Check sheet for the modelled part. Datum: model origin and axes. Units: mm. A direction names the side the tool comes from. Coordinates: 2 decimals unless noted, no trailing zeros. Order: outer loops, then holes, each group sorted by start corner. A loop starts at its lowest first (then second) coordinate and runs counter-clockwise, first axis right, second up.
from build123d import *

# Parameters (mm, degrees)
PAD_DEPTH        = 55.5
HOLE_D           = 4
HOLE_DEPTH       = 25
HOLE_CSINK_D     = 8
HOLE_CSINK_ANGLE = 90
SKETCH002_W      = 3.15
SKETCH002_H      = 24.5
PAD001_DEPTH     = 11.6
CHAMFER_SIZE     = 5
CHAMFER001_SIZE  = 0.5


with BuildPart() as part:
    # Sketch → Pad (new body)
    with BuildSketch(Plane.XZ):
        Polygon((-12.15, 0), (-0.15, 0), (-0.15, 7.65), (11.45, 7.65), (11.45, 11.65), (-12.15, 11.65), align=None)
    extrude(amount=PAD_DEPTH)

    # Hole
    with Locations(Plane(origin=(0, 0, 11.65), x_dir=(-1, 0, 0), z_dir=(0, 0, 1))):
        with Locations((6.15, 10), (6.15, 45.5)):
            CounterSinkHole(HOLE_D / 2, HOLE_CSINK_D / 2, depth=HOLE_DEPTH, counter_sink_angle=HOLE_CSINK_ANGLE)

    # Sketch002 (on Face5 of Hole) → Pad001 (join)
    with BuildSketch(Plane(origin=(-0.15, 0, 0), x_dir=(0, 0, 1), z_dir=(1, 0, 0))):
        with Locations((3.825, 27.75)):
            Rectangle(SKETCH002_W, SKETCH002_H)
    extrude(amount=PAD001_DEPTH)

    # Chamfer
    chamfer_edges = [part.edges().sort_by_distance(p)[0] for p in [
        (11.45, -15.5, 3.825),
        (11.45, -40, 3.825),
    ]]
    chamfer(chamfer_edges, length=CHAMFER_SIZE)

    # Chamfer001
    chamfer001_edges = [part.edges().sort_by_distance(p)[0] for p in [
        (11.45, -27.75, 7.65),
        (11.45, -27.75, 11.65),
        (11.45, 0, 9.65),
        (11.45, -55.5, 9.65),
        (-6.15, -55.5, 0),
        (-0.15, -55.5, 3.825),
        (5.65, -55.5, 7.65),
        (-0.35, -55.5, 11.65),
        (-12.15, -55.5, 5.825),
        (-6.15, 0, 0),
        (-0.15, 0, 3.825),
        (5.65, 0, 7.65),
        (-0.35, 0, 11.65),
        (-12.15, 0, 5.825),
        (-12.15, -27.75, 11.65),
        (-12.15, -27.75, 0),
        (11.45, -27.75, 2.25),
        (11.45, -35, 3.825),
        (11.45, -20.5, 3.825),
        (11.45, -27.75, 5.4),
        (8.95, -18, 2.25),
        (6.45, -15.5, 3.825),
        (8.95, -18, 5.4),
        (8.95, -37.5, 5.4),
        (6.45, -40, 3.825),
        (8.95, -37.5, 2.25),
        (3.15, -40, 2.25),
        (3.15, -40, 5.4),
        (3.15, -15.5, 2.25),
        (3.15, -15.5, 5.4),
        (-0.15, -27.75, 0),
    ]]
    chamfer(chamfer001_edges, length=CHAMFER001_SIZE)


solid = part.part
(1) Tool access check on faces 4 (the flat face through (-0.15, -27, 6)), 5 (the flat face through (3, -40, 4)), 6 (the flat face through (3, -15.5, 4)), 7 (the cylindrical face through (-5.227, -43.726, 4.757)), 8 (the flat face through (8.741, -18.149, 5.154)). Record the directions out of +Z, -Z, +X, -X, +Y, -Y that give a thin tool (end or side, any length) a straight path to the whole face; none if there is none.
Filled in:
face 4: +X
face 5: -Z, +X, -Y
face 6: -Z, +X, +Y
face 7: +Z, -Z
face 8: +X, +Y
(2) Cross-section at B-B (x = 0.75). Enter the section's corners in (y, z), and give its area (3 significant figures).
Filled in:
outline: (-55.5, 8.15) - (-55, 7.65) - (-0.5, 7.65) - (0, 8.15) - (0, 11.15) - (-0.5, 11.65) - (-55, 11.65) - (-55.5, 11.15) - close; (-40, 2.75) - (-39.5, 2.25) - (-16, 2.25) - (-15.5, 2.75) - (-15.5, 4.9) - (-16, 5.4) - (-39.5, 5.4) - (-40, 4.9) - close
area: 298 mm2
(3) Cross-section at C-C (x = -6.15). Enter the section's corners in (y, z), and give its area (3 significant figures).
Filled in:
outline: (-55.5, 0.5) - (-55, 0) - (-47.5, 0) - (-47.5, 9.65) - (-49.5, 11.65) - (-55, 11.65) - (-55.5, 11.15) - close; (-43.5, 0) - (-12, 0) - (-12, 9.65) - (-14, 11.65) - (-41.5, 11.65) - (-43.5, 9.65) - close; (-8, 0) - (-0.5, 0) - (0, 0.5) - (0, 11.15) - (-0.5, 11.65) - (-6, 11.65) - (-8, 9.65) - close
area: 545 mm2
(4) Release check for a two-part mould opening along X. For faces 1 (the flat face through (-6, -27, 0)), 2 (the cylindrical face through (-5.1, -11.7, 4.8)), 3 (the flat face through (8.7, -18.1, 2.5)) record: +X half, -X half, draft (parallel to the pull), parting line (faces both ways), or undercut.
Filled in:
face 1: draft
face 2: undercut
face 3: +X half
(5) Cross-section at D-D (y = -30). Enter the section's corners in (x, z), and give its area (3 significant figures).
Filled in:
outline: (-12.15, 0.5) - (-11.65, 0) - (-0.65, 0) - (-0.15, 0.5) - (-0.15, 2.25) - (10.95, 2.25) - (11.45, 2.75) - (11.45, 4.9) - (10.95, 5.4) - (-0.15, 5.4) - (-0.15, 7.65) - (10.95, 7.65) - (11.45, 8.15) - (11.45, 11.15) - (10.95, 11.65) - (-11.65, 11.65) - (-12.15, 11.15) - close
area: 222 mm2
(6) Thickness scan on probe 1 along Y at (x, z) = (-6.15, 7.75); probe 2 along X at (y, z) = (-10, 2.75). Record the ranges inside material, lowest first.
Filled in:
probe 1: y = -55.5 to -47.5, -43.5 to -12, -8 to 0
probe 2: x = -12.15 to -8.15, -4.15 to -0.15
(7) Go/stop test with flat-tipped pins: P1, Ø8, axis at x = -5.5, y = -25, coming from the -Z side; P2, Ø3, axis at x = -6.15, y = -45.5, coming from the +Z side; P3, Ø5, axis at y = -15.5, z = 4, coming from the +X side; P4, Ø8, axis at x = 6.5, y = -35, coming from the -Z side. Record where each tip stops, or that it passes through.
Filled in:
P1: stops at z = 0
P2: passes through
P3: stops at x = 8.95
P4: stops at z = 2.25
(8) Cross-section at A-A (y = -45.5). Enter the section's corners in (x, z).
Filled in:
outline: (-12.15, 0.5) - (-11.65, 0) - (-8.15, 0) - (-8.15, 9.65) - (-10.15, 11.65) - (-11.65, 11.65) - (-12.15, 11.15) - close; (-4.15, 0) - (-0.65, 0) - (-0.15, 0.5) - (-0.15, 7.65) - (10.95, 7.65) - (11.45, 8.15) - (11.45, 11.15) - (10.95, 11.65) - (-2.15, 11.65) - (-4.15, 9.65) - close
